Verification items for the finished model (mm, model axes). Face numbers are marked on the shaded views. A direction names the side the tool comes from. Give positions to 0.01 mm unless a question says otherwise; leave off trailing zeros. Loops run counter-clockwise (first coordinate to the right, second up) from the corner with the lowest first, then second, coordinate; pieces in that order, holes last. Notation, with made-up numbers: (64, 75) -> (77, 75) arc R25 cw to (77, 88) -> close; hole circle Ø1 at (-24, -32). An arc over 180 degrees is marked (long way). Answer in a Markdown table with one row per item. Add a question column.
Q1. Material ranges on probe 1 along Z at (x, y) = (18, 23); probe 2 along Y at (x, z) = (13, 27.5); probe 3 along X at (y, z) = (3, 25), recorded low to high.
Q2. Section check A-A on x = 0. Enter the section's corners in (y, z), and give its area (3 significant figures).
Q3. Section check C-C on z = 15.5. Enter the section's corners in (x, y), and give its area (3 significant figures).
Q4. Gauge pin test, flat ends, axial feed: P1, Ø2, axis at x = -5.5, z = -2, coming from the -Y side; P2, Ø8, axis at y = -22.5, z = 51, coming from the +X side; P3, Ø8, axis at x = 16.5, z = 6.5, coming from the -Y side. Record the tip position at first contact, or that the pin passes through.
Q5. Set-up check for the marked faces 1 and 2: record each of +Z, -Z, +X, -X, +Y, -Y from which the full face is reachable in a straight line by a thin tool's end or side.
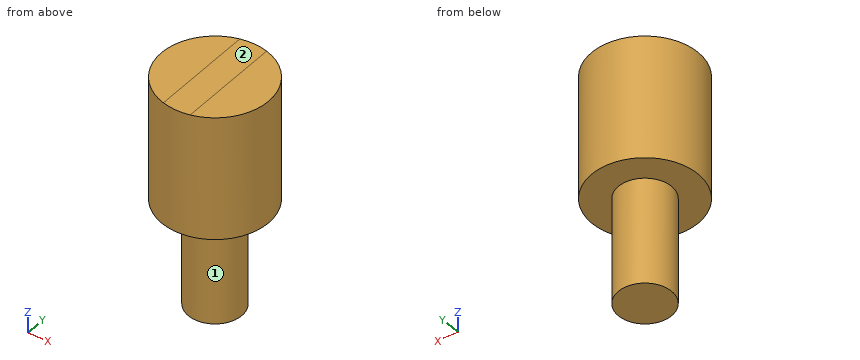
```python
from build123d import *

# Parameters (mm, degrees)
SKETCH1_LINK6_R     = 15
BOSS_EXTRUDE1_DEPTH = 30
SKETCH2_LINK6_R     = 30
BOSS_EXTRUDE2_DEPTH = 69.6
BOSS_EXTRUDE3_DEPTH = 0.001


with BuildPart() as part:
    # sketch1_link6 → Boss-Extrude1 (new body, symmetric)
    with BuildSketch(Plane.XY):
        Circle(SKETCH1_LINK6_R)
    extrude(amount=BOSS_EXTRUDE1_DEPTH, both=True)

    # sketch2_link6 → Boss-Extrude2 (add)
    with BuildSketch(Plane.XY.offset(30)):
        Circle(SKETCH2_LINK6_R)
    extrude(amount=BOSS_EXTRUDE2_DEPTH)

    # sketch3_link6 → Boss-Extrude3 (add)
    with BuildSketch(Plane.XY.offset(99.6)):
        with BuildLine():
            Line((-7.5, 29.047375097), (-7.5, -29.047375097))
            ThreePointArc((-7.5, -29.047375097), (0, -30), (7.5, -29.047375097))
            Line((7.5, -29.047375097), (7.5, 29.047375097))
            ThreePointArc((7.5, 29.047375097), (0, 30), (-7.5, 29.047375097))
        make_face()
    extrude(amount=BOSS_EXTRUDE3_DEPTH)


solid = part.part
```
Taken from the geometry:
| question | item | result |
|---|---|---|
| 1 | probe 1 | z = 30 to 99.6 |
| 1 | probe 2 | y = -7.48 to 7.48 |
| 1 | probe 3 | x = -14.7 to 14.7 |
| 2 | outline | (-30, 30) -> (-15, 30) -> (-15, -30) -> (15, -30) -> (15, 30) -> (30, 30) -> (30, 99.6) -> (-30, 99.6) -> close |
| 2 | area | 5,980 mm² |
| 3 | outline | circle Ø30 at (0, 0) |
| 3 | area | 707 mm² |
| 4 | P1 | stops at y = -14.31 |
| 4 | P2 | stops at x = 23.62 |
| 4 | P3 | stops at y = -8.29 |
| 5 | face 1 | -Z |
| 5 | face 2 | +Z, +X, -X, +Y, -Y |
